from build123d import *

# Parameters (mm, degrees)
F1_DEPTH = 25.4
F2_R     = 16.867449
F3_DEPTH = 25.4
F4_R     = 5.08


with BuildPart() as f1:
    # F0 (on Top) → F1 (new body)
    with BuildSketch(Plane.XY):
        Polygon((57.987113, 61.335813), (0, 61.335813), (-50.072946, 12.33043), (44.593185, 12.33043), align=None)
    extrude(amount=F1_DEPTH)

    # F2 (on face) → F3 (cut)
    with BuildSketch(Plane.XY.offset(25.4)):
        with Locations((25.008492, 42.449769)):
            Circle(F2_R)
    extrude(amount=-F3_DEPTH, mode=Mode.SUBTRACT)

    # F4
    f4_edges = [f1.edges().sort_by_distance(p)[0] for p in [
        (44.593185, 12.33043, 12.7),
        (57.987113, 61.335813, 12.7),
    ]]
    fillet(f4_edges, radius=F4_R)


solid = f1.part
Design review of the part built by this model. Coordinates are the model's own, in mm. Round coordinates to 2 decimals unless told otherwise and drop trailing zeros. Write each loop counter-clockwise with the first axis right and the second up, starting at its lowest first coordinate (ties: lowest second). Pieces come first, ordered by that corner, then holes. Notation, with made-up numbers: M 23,-24.75 L 63,-24.75 A26 cw 63,-2.75 Z; hole C 40,48 d1. An arc over 180 degrees is marked long. One line per item, written item: value. Start each with the question number.
1. Clearance check with flat-ended pins moving along their axes: P1, Ø4, axis at y = 25.5, z = 19, coming from the +X side; P2, Ø6, axis at y = 56, z = 6, coming from the -X side; P3, Ø6, axis at y = 24.5, z = 21, coming from the -X side. State where each tip first meets the part, or that it passes through.
2. Take a section at B-B on x = 34.5. State the section outline as (y, z) points, then the cut area to 3 significant figures.
3. Take a section at D-D on y = 18. State the section outline as (x, z) points.
4. Take a section at C-C on z = 11. State the section outline as (x, y) points, then the cut area to 3 significant figures.
5. Draft analysis for pull direction X (two halves, no side actions). For faces 1 (the face through (2, 32, 0)), 2 (the face through (22.813, 59.174, 12.878)), 3 (the face through (43.834, 13.401, 12.878)), state which applies: pulls with the +X half, pulls with the -X half, needs draft (parallel to the pull), parting line crosses it, or undercut.
6. Take a section at A-A on y = 51. State the section outline as (x, z) points, then the cut area to 3 significant figures.
7. To check wall thickness, follow probe 1 along X at (y, z) = (51, 22.5); probe 2 along X at (y, z) = (31.5, 15.75); probe 3 along Y at (x, z) = (17, 23.75). State the ranges of each line that lie inside material, in increasing order. Write a range as from..to.
Computed:
1. P1: stops at x = 48.74
1. P2: stops at x = -8.52
1. P3: stops at x = -40.7
2. outline: M 12.33,0 L 28.51,0 L 28.51,25.4 L 12.33,25.4 Z; M 56.39,0 L 61.34,0 L 61.34,25.4 L 56.39,25.4 Z
2. area: 536 mm²
3. outline: M -44.28,0 L 46.14,0 L 46.14,25.4 L -44.28,25.4 Z
4. outline: M -50.07,12.33 L 40.72,12.33 A5.08 ccw 45.62,16.07 L 56.23,54.92 A5.08 ccw 51.33,61.34 L 0,61.34 Z; hole C 25.01,42.45 d33.73
4. area: 2,830 mm²
5. face 1: needs draft
5. face 2: undercut
5. face 3: pulls with the +X half
6. outline: M -10.56,0 L 10.47,0 L 10.47,25.4 L -10.56,25.4 Z; M 39.55,0 L 55.16,0 L 55.16,25.4 L 39.55,25.4 Z
6. area: 931 mm²
7. probe 1: x = -10.56..10.47, 39.55..55.16
7. probe 2: x = -30.49..12.18, 37.84..49.83
7. probe 3: y = 12.33..27.6, 57.29..61.34
